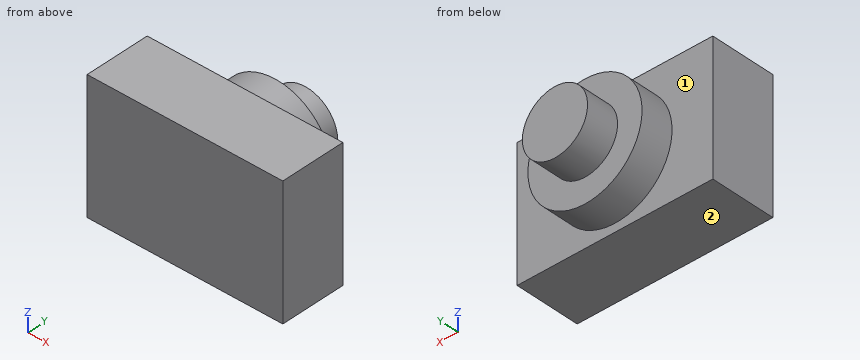
from build123d import *

# Parameters (mm, degrees)
SKETCH008_W             = 12
SKETCH008_H             = 8
PAD006_DEPTH            = 4
SKETCH009_R             = 3.5
PAD007_DEPTH            = 2
SKETCH010_R             = 2
PAD008_DEPTH            = 2
BODY002_PLACEMENT_ANGLE = 90


with BuildPart() as part:
    # Sketch008 → Pad006 (new body)
    with BuildSketch(Plane.XY):
        Rectangle(SKETCH008_W, SKETCH008_H)
    extrude(amount=PAD006_DEPTH)

    # Sketch009 (on Face5 of Pad006) → Pad007 (join)
    with BuildSketch(Plane(origin=(0, 0, 0), x_dir=(1, 0, 0), z_dir=(0, 0, -1))):
        Circle(SKETCH009_R)
    extrude(amount=PAD007_DEPTH)

    # Sketch010 (on Face8 of Pad007) → Pad008 (join)
    with BuildSketch(Plane(origin=(0, 0, -2), x_dir=(1, 0, 0), z_dir=(0, 0, -1))):
        Circle(SKETCH010_R)
    extrude(amount=PAD008_DEPTH)


with BuildPart() as part_1:
    # Body002 placement: moved
    add(part.part.moved(Location((0, 30.2, 16))).rotate(Axis((0, 30.2, 16), (1, 0, 0)), BODY002_PLACEMENT_ANGLE))


solid = part_1.part
Could you check a few things on this model? Use its own coordinates, in mm. Face numbers are marked on the shaded views. A direction names the side the tool comes from. Give positions to 0.01 mm unless a question says otherwise; leave off trailing zeros. Order: outer loops, then holes, each group sorted by start corner. A loop starts at its lowest first (then second) coordinate and runs counter-clockwise, first axis right, second up.
Item 1: For the marked faces 1 and 2, which set-ups out of +Z, -Z, +X, -X, +Y, -Y let a thin tool reach every point of the face, with its end or its side?
Item 2: If we section it at A-A, the plane x = 0: Write out the boundary of the cut face in (y, z), plus the area to 3 significant figures.
Item 3: If we section it at B-B, the plane z = 16: Write out the boundary of the cut face in (x, y), plus the area to 3 significant figures.
Item 4: If we section it at C-C, the plane y = 32.5: Write out the boundary of the cut face in (x, z).
Item 5: I need wall thicknesses on line 1 (Y direction, x = -1.75, z = 13.5); line 2 (Y direction, x = -4, z = 14.25); line 3 (X direction, y = 31.25, z = 16.75). Which ranges of each line are inside material? Lowest first, please.
Item 6: If we section it at D-D, the plane x = 2.25: Write out the boundary of the cut face in (y, z), plus the area to 3 significant figures.
Item 7: I'm going to push a flat-ended pin straight in: pin 1 (1 mm diameter, centred on x = 4.5, z = 18, fed in from +Y). Where does the tip first touch, or does it pass through?
Values:
1. face 1: +Y
1. face 2: -Z, +X, -X, +Y, -Y
2. outline: (26.2, 12) - (30.2, 12) - (30.2, 12.5) - (32.2, 12.5) - (32.2, 14) - (34.2, 14) - (34.2, 18) - (32.2, 18) - (32.2, 19.5) - (30.2, 19.5) - (30.2, 20) - (26.2, 20) - close
2. area: 54.0 mm2
3. outline: (-6, 26.2) - (6, 26.2) - (6, 30.2) - (3.5, 30.2) - (3.5, 32.2) - (2, 32.2) - (2, 34.2) - (-2, 34.2) - (-2, 32.2) - (-3.5, 32.2) - (-3.5, 30.2) - (-6, 30.2) - close
3. area: 70.0 mm2
4. outline: circle Ø4 at (0, 16)
5. line 1: y = 26.2 to 32.2
5. line 2: y = 26.2 to 30.2
5. line 3: x = -3.42 to 3.42
6. outline: (26.2, 12) - (30.2, 12) - (30.2, 13.32) - (32.2, 13.32) - (32.2, 18.68) - (30.2, 18.68) - (30.2, 20) - (26.2, 20) - close
6. area: 42.7 mm2
7. pin 1: stops at y = 30.2
